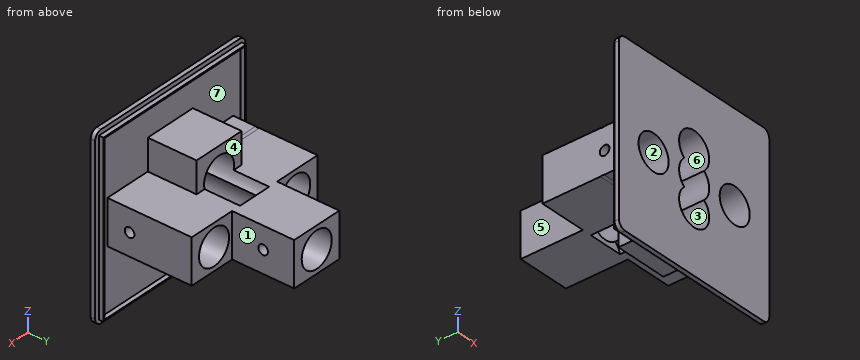
```python
from build123d import *

# Parameters (mm, degrees)
SKETCH1_W                       = 19.05
SKETCH1_H                       = 19.05
BOSS_EXTRUDE1_DEPTH             = 38.1
SKETCH6_W                       = 19.05
SKETCH6_H                       = 15.875
BOSS_EXTRUDE3_DEPTH             = 34.925
SKETCH2_R                       = 6.35
CUT_EXTRUDE1_DEPTH              = 31.75
SKETCH8_R                       = 6.35
CUT_EXTRUDE4_DEPTH              = 67.750552432
SKETCH10_W                      = 17.05
SKETCH10_H                      = 15.875
BOSS_EXTRUDE4_DEPTH             = 31.75
SKETCH11_R                      = 6.35
CUT_EXTRUDE6_DEPTH              = 31.75
CUT_EXTRUDE7_REACH              = 70.78
CUT_EXTRUDE7_END_RADIUS         = 6.35
SKETCH12_R                      = 1.7272
SKETCH13_W                      = 63.5
SKETCH13_H                      = 63.5
BOSS_EXTRUDE5_DEPTH             = 1.5875
CUT_EXTRUDE9_REACH              = 81.121
CUT_EXTRUDE9_END_RADIUS         = 6.35
SKETCH15_R                      = 1.7272
SKETCH16_W                      = 60.325
SKETCH16_H                      = 60.325
SKETCH16_W_2                    = 59.425
SKETCH16_H_2                    = 59.425
BOSS_EXTRUDE6_DEPTH             = 1.5875
FILLET1_R                       = 2.54
CUT_EXTRUDE10_REACH             = 81.121
SKETCH18_R                      = 1.7272
CUT_EXTRUDE10_DIRECTION_2_DEPTH = 80.12059235


with BuildPart() as part:
    # Sketch1 → Boss-Extrude1 (new body)
    with BuildSketch(Plane.XY):
        Rectangle(SKETCH1_W, SKETCH1_H)
    extrude(amount=BOSS_EXTRUDE1_DEPTH)

    # Sketch6 → Boss-Extrude3 (add)
    with BuildSketch(Plane(origin=(0, 9.525, 0), x_dir=(1, 0, 0), z_dir=(0, 1, 0))):
        with Locations((0, -19.05)):
            Rectangle(SKETCH6_W, SKETCH6_H)
    extrude(amount=BOSS_EXTRUDE3_DEPTH)

    # Sketch2 → Cut-Extrude1 (cut)
    with BuildSketch(Plane(origin=(0, -9.525, 0), x_dir=(-1, 0, 0), z_dir=(0, -1, 0))):
        with Locations(Location((0, -28.575, 0), (0, 0, 90))):
            Circle(SKETCH2_R)
        with Locations(Location((0, -9.525, 0), (0, 0, 90))):
            Circle(SKETCH2_R)
    extrude(amount=-CUT_EXTRUDE1_DEPTH, mode=Mode.SUBTRACT)

    # Sketch8 → Cut-Extrude4 (cut, through all)
    with BuildSketch(Plane(origin=(0, 44.45, 0), x_dir=(1, 0, 0), z_dir=(0, 1, 0))):
        with Locations(Location((0, -19.05, 0), (0, 0, 270))):
            Circle(SKETCH8_R)
    extrude(amount=-CUT_EXTRUDE4_DEPTH, mode=Mode.SUBTRACT)

    # Sketch10 → Boss-Extrude4 (add)
    with BuildSketch(Plane(origin=(0, -9.525, 0), x_dir=(-1, 0, 0), z_dir=(0, -1, 0))):
        with Locations((-18.05, -19.05)):
            Rectangle(SKETCH10_W, SKETCH10_H)
    boss_extrude4 = extrude(amount=-BOSS_EXTRUDE4_DEPTH)

    # Sketch11 → Cut-Extrude6 (cut)
    with BuildSketch(Plane(origin=(0, -9.525, 0), x_dir=(-1, 0, 0), z_dir=(0, -1, 0))):
        with Locations(Location((-17.145, -19.05, 0), (0, 0, 90))):
            Circle(SKETCH11_R)
    cut_extrude6 = extrude(amount=-CUT_EXTRUDE6_DEPTH, mode=Mode.SUBTRACT)

    # Cut-Extrude7: up to this cylinder (the profile starts outside it)
    cut_extrude7_end = Plane(origin=(17.145, 0, 19.05), z_dir=(0, -1, 0)) * Cylinder(CUT_EXTRUDE7_END_RADIUS, 155.26, mode=Mode.PRIVATE)
    # Sketch12 → Cut-Extrude7 (cut, up to the surface)
    with BuildSketch(Plane(origin=(26.575, 0, 0), x_dir=(0, 0, -1), z_dir=(1, 0, 0)), mode=Mode.PRIVATE) as cut_extrude7_sk1:
        with Locations((-19.05, 0)):
            Circle(SKETCH12_R)
    cut_extrude7_tool1 = extrude(cut_extrude7_sk1.sketch, amount=-CUT_EXTRUDE7_REACH, mode=Mode.PRIVATE) - cut_extrude7_end
    cut_extrude7 = cut_extrude7_tool1.solids().sort_by_distance((26.575, 0, 19.05))[0]
    add(cut_extrude7, mode=Mode.SUBTRACT)

    # Mirror1: Boss-Extrude4, Cut-Extrude6, Cut-Extrude7 across plane
    add(boss_extrude4.mirror(Plane(origin=(0, 0, 0), x_dir=(0, 0, 1), z_dir=(1, 0, 0))))
    add(cut_extrude6.mirror(Plane(origin=(0, 0, 0), x_dir=(0, 0, 1), z_dir=(1, 0, 0))), mode=Mode.SUBTRACT)
    add(cut_extrude7.mirror(Plane(origin=(0, 0, 0), x_dir=(0, 0, 1), z_dir=(1, 0, 0))), mode=Mode.SUBTRACT)

    # Sketch13 → Boss-Extrude5 (add)
    with BuildSketch(Plane(origin=(0, -9.525, 0), x_dir=(-1, 0, 0), z_dir=(0, -1, 0))):
        with Locations((0, -19.05)):
            Rectangle(SKETCH13_W, SKETCH13_H)
        Polygon((9.525, -26.9875), (26.575, -26.9875), (26.575, -11.1125), (9.525, -11.1125), (9.525, 0), (-9.525, 0), (-9.525, -11.1125), (-26.575, -11.1125), (-26.575, -26.9875), (-9.525, -26.9875), (-9.525, -38.1), (9.525, -38.1), align=None, mode=Mode.SUBTRACT)
    extrude(amount=-BOSS_EXTRUDE5_DEPTH)

    # Cut-Extrude9: up to this cylinder (the profile starts outside it)
    cut_extrude9_end = Plane(origin=(0, 33.3375, 19.05), z_dir=(0, 1, 0)) * Cylinder(CUT_EXTRUDE9_END_RADIUS, 175.942, mode=Mode.PRIVATE)
    # Sketch15 → Cut-Extrude9 (cut, up to the surface)
    with BuildSketch(Plane(origin=(9.525, 0, 0), x_dir=(0, 0, -1), z_dir=(1, 0, 0)), mode=Mode.PRIVATE) as cut_extrude9_sk1:
        with Locations((-19.05, 33.3375)):
            Circle(SKETCH15_R)
    cut_extrude9_tool1 = extrude(cut_extrude9_sk1.sketch, amount=-CUT_EXTRUDE9_REACH, mode=Mode.PRIVATE) - cut_extrude9_end
    add(cut_extrude9_tool1.solids().sort_by_distance((9.525, 33.3375, 19.05))[0], mode=Mode.SUBTRACT)

    # Sketch16 → Boss-Extrude6 (add)
    with BuildSketch(Plane(origin=(0, -7.9375, 0), x_dir=(1, 0, 0), z_dir=(0, 1, 0))):
        with Locations((0, -19.05)):
            Rectangle(SKETCH16_W, SKETCH16_H)
        with Locations((0, -19.05)):
            Rectangle(SKETCH16_W_2, SKETCH16_H_2, mode=Mode.SUBTRACT)
    extrude(amount=BOSS_EXTRUDE6_DEPTH)

    # Fillet1
    fillet1_edges = [part.edges().sort_by_distance(p)[0] for p in [
        (31.75, -8.73125, 50.8),
        (31.75, -8.73125, -12.7),
        (-31.75, -8.73125, -12.7),
        (-31.75, -8.73125, 50.8),
    ]]
    fillet(fillet1_edges, radius=FILLET1_R)

    # Sketch18 → Cut-Extrude10 (cut, up to next)
    with BuildSketch(Plane.ZY.offset(9.525), mode=Mode.PRIVATE) as cut_extrude10_sk1:
        with Locations(Location((28.575, 0.79375, 0), (0, 0, 156.797426943))):
            Circle(SKETCH18_R)
    cut_extrude10_tool1 = extrude(cut_extrude10_sk1.sketch, amount=-CUT_EXTRUDE10_REACH, mode=Mode.PRIVATE) & part.part
    # Sketch18 → Cut-Extrude10 (cut, up to next)
    with BuildSketch(Plane.ZY.offset(9.525), mode=Mode.PRIVATE) as cut_extrude10_sk2:
        with Locations(Location((9.525, 0.79375, 0), (0, 0, 336.797426943))):
            Circle(SKETCH18_R)
    cut_extrude10_tool2 = extrude(cut_extrude10_sk2.sketch, amount=-CUT_EXTRUDE10_REACH, mode=Mode.PRIVATE) & part.part
    add(cut_extrude10_tool1.solids().sort_by_distance((-9.525, 0.79375, 28.575))[0], mode=Mode.SUBTRACT)
    add(cut_extrude10_tool2.solids().sort_by_distance((-9.525, 0.79375, 9.525))[0], mode=Mode.SUBTRACT)

    # Sketch18 → Cut-Extrude10 direction 2 (cut)
    with BuildSketch(Plane.ZY.offset(9.525)):
        with Locations(Location((28.575, 0.79375, 0), (0, 0, 156.797426943))):
            Circle(SKETCH18_R)
        with Locations(Location((9.525, 0.79375, 0), (0, 0, 336.797426943))):
            Circle(SKETCH18_R)
    extrude(amount=CUT_EXTRUDE10_DIRECTION_2_DEPTH, mode=Mode.SUBTRACT)


solid = part.part
```
Build history of the part. All positions in model axes, mm. Face numbers are marked on the shaded views. A direction names the side the tool comes from. Give positions to 0.01 mm unless a question says otherwise; leave off trailing zeros. Return JSON: item names as keys, results as strings.
Q1. Band-saw the part on A-A (y = 20.5). Count the separate pieces of the cut face and the enclosed holes in it, then the cut area to 3 significant figures.
Answer list:
{"separate pieces": "2", "enclosed holes": "2", "area": "414 mm^2"}
Q2. Flat gauge pins, fed straight in: pin 1 (0.5 mm diameter, centred on x = 7.5, y = -7, fed in from +Z); pin 2 (1.5 mm diameter, centred on y = 28.5, z = 16.5, fed in from -X) (3 decimals); pin 3 (1.3 mm diameter, centred on x = -2.5, y = -7, fed in from -Z). Where does each tip first touch, or does it go through?
Answer list:
{"pin 1": "stops at z = 49.21", "pin 2": "stops at x = -9.525", "pin 3": "stops at z = -11.11"}
Q3. Two-plate mould, pull along X, no slides. Class the marked faces 4, 5, 6 and 7: pulls with the +X half, pulls with the -X half, needs draft (parallel to the pull), parting line crosses it, or undercut.
Answer list:
{"face 4": "needs draft", "face 5": "pulls with the -X half", "face 6": "undercut", "face 7": "undercut"}
Q4. 3-axis set-ups, long thin cutter, end or side, ignore diameter. For the marked faces 1, 2 and 3: which of +Z, -Z, +X, -X, +Y, -Y reach the whole face in a straight line?
Answer list:
{"face 1": "+Z, -Z, +X, +Y", "face 2": "+Y, -Y", "face 3": "-Y"}
Q5. Wall check: probe 1 along Y at (x, z) = (8.2, 19.05) (3 decimals); probe 2 along X at (y, z) = (-1.5, 9.5) (3 decimals); probe 3 along Z at (x, y) = (-5, -6). Give the ranges that are in metal, low to high. Write a range as from..to.
Answer list:
{"probe 1": "y = -9.525..31.61, 35.065..44.45", "probe 2": "x = -9.525..-6.35, 6.35..9.525", "probe 3": "z = 0..5.61, 13.44..15.14, 22.96..24.66, 32.49..38.1"}
